Autodesk Inventor part; units mm, degrees
ref_plane "YZ Plane" through (0, 0, 0) normal (1, 0, 0) x (0, 1, 0)
ref_plane "XZ Plane" through (0, 0, 0) normal (0, 1, 0) x (-1, 0, 0)
ref_plane "XY Plane" through (0, 0, 0) normal (0, 0, 1) x (1, 0, 0)
sketch "Эскиз1" plane through (0, 0, 0) normal (0, 0, 1) x (1, 0, 0)
  line L0 (-38, 52.38) -> (38, 52.38) construction
  line L1 (38, 52.38) -> (38, -52.38) construction
  line L2 (38, -52.38) -> (-38, -52.38) construction
  line L3 (-38, -52.38) -> (-38, 52.38) construction
  line L4 (-26.6205, -33.05) -> (26.6205, -33.05) construction
  line L5 (26.6205, -33.05) -> (26.6205, 33.05) construction
  line L6 (26.6205, 33.05) -> (-26.6205, 33.05) construction
  line L7 (-26.6205, 33.05) -> (-26.6205, -33.05) construction
  line L8 (0, 33.05) -> (0, 38.05) construction
  line L9 (0, -33.05) -> (0, -38.05) construction
  line L10 (-38, 38.05) -> (38, 38.05)
  line L11 (38, 38.05) -> (38, -38.05)
  line L12 (38, -38.05) -> (-38, -38.05)
  line L13 (-38, -38.05) -> (-38, 38.05)
  dimension "d0" = 76
  dimension "d1" = 104.76
  dimension "d2" = 53.241
  dimension "d3" = 66.1
  dimension "d4" = 5
  dimension "d5" = 5
extrude "Выдавливание1" add sketch "Эскиз1" along normal blind 5
sketch "Эскиз2" plane through (0, 0, 5) normal (0, 0, 1) x (1, 0, 0)
  line L0 (38, 38.05) -> (38, -38.05)
  line L1 (-38, -38.05) -> (-38, 38.05)
  line L2 (-38, 38.05) -> (-38, -38.05)
  line L3 (-38, -38.05) -> (-42, -38.05)
  line L4 (38, 38.05) -> (42, 38.05)
  line L5 (42, -38.05) -> (42, 38.05)
  line L6 (-42, 38.05) -> (-42, -38.05)
  line L7 (-38, -38.05) -> (-38, 38.05)
  line L8 (38, 38.05) -> (-38, 38.05)
  line L9 (38, 38.05) -> (38, -38.05)
  line L10 (42, 38.05) -> (38, 38.05)
  line L11 (-38, 38.05) -> (-42, 38.05)
  line L12 (-42, -38.05) -> (-38, -38.05)
  line L13 (38, -38.05) -> (42, -38.05)
  point P0 (0, 0)
  dimension "d8" = 4
  dimension "d9" = 4
extrude "Выдавливание2" add sketch "Эскиз2" along normal blind 24 and the other way blind 5
sketch "Эскиз3" plane through (0, 0, 29) normal (0, 0, 1) x (1, 0, 0)
  line L0 (38, 38.05) -> (38, -38.05)
  line L1 (38, -38.05) -> (42, -38.05)
  line L2 (42, -38.05) -> (42, 38.05)
  line L3 (42, 38.05) -> (38, 38.05)
  line L4 (42, 9.5) -> (38, 9.5)
  line L5 (38, 9.5) -> (38, -9.5)
  line L6 (38, -9.5) -> (42, -9.5)
  line L7 (42, -9.5) -> (42, 9.5)
  line L8 (42, 9.5) -> (38, -9.5) construction
  line L9 (38, 9.5) -> (42, -9.5) construction
  line L10 (0, 0) -> (0, -84) construction
  line L11 (-42, 9.5) -> (-38, 9.5)
  line L12 (-38, -9.5) -> (-42, -9.5)
  line L13 (-38, 9.5) -> (-38, -9.5) construction
  line L14 (-38, 38.05) -> (-38, -38.05) construction
  line L15 (-42, 9.5) -> (-42, -9.5) construction
  line L16 (-42, 38.05) -> (-42, -38.05) construction
  line L17 (-38, 9.5) -> (-38, -9.5)
  line L18 (-42, -9.5) -> (-42, 9.5)
  point P0 (40, 0)
  dimension "d14" = 4
  dimension "d15" = 19
extrude "Выдавливание3" cut sketch "Эскиз3" against normal up to surface (24 mm away) contours L4 L2 L6 L0 | L11 L17 L12 L18
sketch "Эскиз4" plane through (-42, 38.05, 0) normal (0, 1, 0) x (1, 0, 0)
  line L0 (0, 0) -> (84, 0)
  line L1 (0, 0) -> (0, -29)
  line L2 (4, -29) -> (0, -29)
  line L3 (4, -29) -> (4, -5)
  line L4 (80, -5) -> (4, -5)
  line L5 (80, -29) -> (80, -5)
  line L6 (84, -29) -> (80, -29)
  line L7 (84, 0) -> (84, -29)
  point P0 (42, 0)
extrude "Выдавливание4" cut sketch "Эскиз4" against normal blind 29
sketch "Эскиз5" plane through (0, 0, 29) normal (0, 0, 1) x (1, 0, 0)
  line L0 (-38, -9.5) -> (-42, -9.5)
  line L1 (-42, -9.5) -> (-42, -38.05)
  line L2 (-42, -38.05) -> (-38, -38.05)
  line L3 (-38, -38.05) -> (-38, -9.5)
  line L4 (42, -9.5) -> (38, -9.5)
  line L5 (38, -9.5) -> (38, -38.05)
  line L6 (38, -38.05) -> (42, -38.05)
  line L7 (42, -38.05) -> (42, -9.5)
  point P0 (0, 0)
extrude "Выдавливание5" add sketch "Эскиз5" along normal blind 12
properties part number "Ard for BR"
Verification items for the finished model (mm, model axes). A direction names the side the tool comes from. Give positions to 0.01 mm unless a question says otherwise; leave off trailing zeros. Loops run counter-clockwise (first coordinate to the right, second up) from the corner with the lowest first, then second, coordinate; pieces in that order, holes last. Notation, with made-up numbers: M -24,-27 L 18,-27 A5 ccw 18,-19 Z; hole C 65,84 d8. An arc over 180 degrees is marked long. Return JSON: item names as keys, results as strings.
1) Section check A-A, the plane z = 27.5. Enter the section's corners in (x, y), and give its area (3 significant figures).
Findings:
{"outline": "M -42,-38.05 L -38,-38.05 L -38,-9.5 L -42,-9.5 Z; M 38,-38.05 L 42,-38.05 L 42,-9.5 L 38,-9.5 Z", "area": "228 mm2"}
2) Tool access check on faces 1 (the flat face through (42, -20, 20)), 2 (the flat face through (40, -9.5, 23)), 3 (the flat face through (-38, -24, 23)). Record the directions out of +Z, -Z, +X, -X, +Y, -Y that give a thin tool (end or side, any length) a straight path to the whole face; none if there is none.
Findings:
{"face 1": "+Z, -Z, +X, +Y, -Y", "face 2": "+Z, +X, -X, +Y", "face 3": "+Z, +Y, -Y"}
3) Material ranges on L1, parallel to X at y = -15, z = 35; L2, parallel to Z at x = -12, y = -33.5, recorded low to high. Write a range as [from, to].
Findings:
{"L1": "x = [-42, -38], [38, 42]", "L2": "z = [0, 5]"}
4) Section check C-C, the plane x = -1.5. Enter the section's corners in (y, z).
Findings:
{"outline": "M -38.05,0 L 9.05,0 L 9.05,5 L -38.05,5 Z"}
5) Gauge pin test, flat ends, axial feed: P1, Ø4.5, axis at x = -39.5, z = 26, coming from the +Y side; P2, Ø1, axis at x = -9, y = -9.5, coming from the +Z side. Record the tip position at first contact, or that the pin passes through.
Findings:
{"P1": "stops at y = -9.5", "P2": "stops at z = 5"}
6) Mould release check, pull along X, two halves, no side actions. Record for faces 4 (the flat face through (40, -24, 41)), 5 (the flat face through (38, -24, 23)), 6 (the flat face through (-42, -25, 20)): released by +X, released by -X, zero draft, split by the parting line, or undercut.
Findings:
{"face 4": "zero draft", "face 5": "undercut", "face 6": "released by -X"}
7) Section check B-B, the plane y = -11. Enter the section's corners in (x, z).
Findings:
{"outline": "M -42,0 L 42,0 L 42,41 L 38,41 L 38,5 L -38,5 L -38,41 L -42,41 Z"}
8) Section check D-D, the plane y = -1.5. Enter the section's corners in (x, z).
Findings:
{"outline": "M -42,0 L 42,0 L 42,5 L -42,5 Z"}
